Design review of the part built by this model. Coordinates are the model's own, in mm. Coordinates: 2 decimals unless noted, no trailing zeros. Loops run counter-clockwise (first coordinate to the right, second up) from the corner with the lowest first, then second, coordinate; pieces in that order, holes last. Notation, with made-up numbers: (30, 30) -> (79, 30) arc R20 cw to (79, 62) -> close; hole circle Ø9 at (58, 7.5). An arc over 180 degrees is marked (long way). Answer as a JSON object with one key per item and string values.
```python
from build123d import *

# Parameters (mm, degrees)
SKETCH1_R           = 12.2
BOSS_EXTRUDE1_DEPTH = 16
SKETCH3_R           = 11.5
CUT_EXTRUDE1_DEPTH  = 15
CUT_EXTRUDE2_START  = -0.2
SKETCH2_R           = 12.2
SKETCH2_R_2         = 11.65
CUT_EXTRUDE2_DEPTH  = 0.2


with BuildPart() as part:
    # Sketch1 → Boss-Extrude1 (new body)
    with BuildSketch(Plane.XY):
        Circle(SKETCH1_R)
    extrude(amount=BOSS_EXTRUDE1_DEPTH)

    # Sketch3 → Cut-Extrude1 (cut)
    with BuildSketch(Plane.XY.offset(16)):
        Circle(SKETCH3_R)
    extrude(amount=-CUT_EXTRUDE1_DEPTH, mode=Mode.SUBTRACT)

    # Sketch2 → Cut-Extrude2 (cut)
    with BuildSketch(Plane.XY.offset(16).offset(CUT_EXTRUDE2_START)):
        Circle(SKETCH2_R)
        Circle(SKETCH2_R_2, mode=Mode.SUBTRACT)
    extrude(amount=CUT_EXTRUDE2_DEPTH, mode=Mode.SUBTRACT)


solid = part.part
```
1) Clearance check with flat-ended pins moving along their axes: pin 1 Ø1 at (x, y) = (-6, 7) entering from +Z; pin 2 Ø8 at (y, z) = (-3.5, 7.5) entering from -X; pin 3 Ø6 at (x, z) = (3.5, 3.5) entering from +Y; pin 4 Ø3 at (x, z) = (-5, 11.5) entering from -Y. State where each tip first meets the part, or that it passes through.
Completed:
{"pin 1": "z = 1", "pin 2": "x = -12.2", "pin 3": "y = 12.19", "pin 4": "y = -11.69"}
2) Add section C-C, the plane z = 10.25. Give the boundary of the cut face in (x, y).
Completed:
{"outline": "circle Ø24.4 at (0, 0); hole circle Ø23 at (0, 0)"}
3) The part is to be moulded in two halves that separate along X. For faces 1 (the flat face through (0, 0, 1)), 2 (the flat face through (0, 0, 0)), 3 (the cylindrical face through (-12.19, 0.54, 7.79)), say which applies: pulls with the +X half, pulls with the -X half, needs draft (parallel to the pull), parting line crosses it, or undercut.
Completed:
{"face 1": "undercut", "face 2": "needs draft", "face 3": "parting line crosses it"}
4) Add section A-A, the plane y = 0. Give the boundary of the cut face in (x, z), and give its area (3 significant figures).
Completed:
{"outline": "(-12.2, 0) -> (12.2, 0) -> (12.2, 15.8) -> (11.65, 15.8) -> (11.65, 16) -> (11.5, 16) -> (11.5, 1) -> (-11.5, 1) -> (-11.5, 16) -> (-11.65, 16) -> (-11.65, 15.8) -> (-12.2, 15.8) -> close", "area": "45.2 mm²"}
5) Wall thickness on probe 1 along Y at (x, z) = (0, 7.5); probe 2 along Z at (x, y) = (7.5, -1): over which ranges is each line inside the solid? List them lowest first.
Completed:
{"probe 1": "-12.2 to -11.5, 11.5 to 12.2", "probe 2": "0 to 1"}
